The model under review builds one solid part; all positions refer to its coordinate system, in mm. A direction names the side the tool comes from. Coordinates: 2 decimals unless noted, no trailing zeros. Write each loop counter-clockwise with the first axis right and the second up, starting at its lowest first coordinate (ties: lowest second). Pieces come first, ordered by that corner, then holes. Notation, with made-up numbers: (47.5, 41) - (105.5, 41) arc R26 ccw to (105.5, 58) - close; hole circle Ø6 at (6, 86). An arc over 180 degrees is marked (long way). Return JSON: item names as keys, results as strings. Group by question number.
(1) Tool access review of faces 1 (the face through (-166.436, -12.522, 21.226)), 2 (the face through (-129, 0, 21)), 3 (the face through (-130, 0, 4)): name each direction out of +Z, -Z, +X, -X, +Y, -Y from which nothing blocks a thin tool from reaching the whole face with its end or side.
(2) To check wall thickness, follow L1, parallel to Y at x = 182, z = 10.75; L2, parallel to X at y = -7.5, z = 16.5; L3, parallel to X at y = 20, z = 4.75. State the ranges of each line that lie inside material, in increasing order. Write a range as from..to.
(3) We need section A-A on y = 12.7. State the section outline as (x, z) points.
(4) For pin 1 Ø20.5 at (x, y) = (-134, -14) entering from -Z; pin 2 Ø6 at (y, z) = (0.5, 16) entering from -X; pin 3 Ø7.5 at (x, z) = (191.5, 15) entering from -Y; pin 4 Ø5 at (x, z) = (196.67, 4.57) entering from +Y, all flat-tipped, find the tip position at first contact; note any pin that passes through.
(5) We need section C-C on y = -12.7. Give the number of separate pieces and of enclosed holes in the cut face, then the cut area to 3 significant figures.
(6) Draft analysis for pull direction Z (two halves, no side actions). For faces 4 (the face through (171.6, 12.8, 12.5)), 5 (the face through (-18, 0, 0)), 6 (the face through (-16, -25.4, 13)), 7 (the face through (-205, 0, 8.467)), state which applies: released by +Z, released by -Z, zero draft, split by the parting line, or undercut.
(7) We need section B-B on x = -136. State the section outline as (y, z) points.
```python
from build123d import *

# Parameters (mm, degrees)
F1_DEPTH  = 25.4
F3_DEPTH  = 8.4666666667
F5_DEPTH  = 8.4666666667
F6_W      = 25.4
F6_H      = 8.4666666667
F9_W      = 27.051
F9_H      = 8.4666666667
F13_R     = 6.35
F14_DEPTH = 16.9343333333
F12_R     = 3.175
F15_DEPTH = 42.3343333333
F16_R     = 6.35
F17_DEPTH = 25.401


with BuildPart() as f1:
    # F0 (on Top) → F1 (new body)
    with BuildSketch(Plane.XY):
        Polygon((-232.5293936748, 25.4), (-203.2, -25.4), (203.2, -25.4), (203.2, 25.4), align=None)
    extrude(amount=F1_DEPTH)

    # F2 (on face) → F3 (cut)
    with BuildSketch(Plane.XY.offset(25.4)):
        Polygon((-159.2059094878, 0), (-173.8706063252, -25.4), (-115.2118189755, -25.4), (-100.5471221381, 0), align=None)
    extrude(amount=-F3_DEPTH, mode=Mode.SUBTRACT)

    # F4 (on face) → F5 (cut)
    with BuildSketch(Plane(origin=(0, 0, 0), x_dir=(1, 0, 0), z_dir=(0, 0, -1))):
        Polygon((-100.5471221381, 0), (-115.2118189755, 25.4), (-173.8706063252, 25.4), (-159.2059094878, 0), align=None)
    extrude(amount=-F5_DEPTH, mode=Mode.SUBTRACT)

    # F7: sweep along a path in F7_path
    with BuildLine(Plane(origin=(-232.5293936748, 25.4, 25.4), x_dir=(-0.5, 0.8660254038, 0), z_dir=(-0.8660254038, -0.5, 0))) as f7_path:
        Line((0, 0), (-58.6587873497, 0))
    # F6 (on face) → F7 (sweep, cut)
    with BuildSketch(Plane(origin=(0, 25.4, 0), x_dir=(-1, 0, 0), z_dir=(0, 1, 0))):
        with Locations((219.8293936748, 12.7)):
            Rectangle(F6_W, F6_H)
    sweep(path=f7_path.line, mode=Mode.SUBTRACT)

    # F10: sweep along a path in F8
    with BuildLine(Plane.XZ.offset(25.4)) as f10_path:
        Line((193.9551560496, 25.4), (203.2, 0))
    # F9 (on face) → F10 (sweep, cut)
    with BuildSketch(Plane.XY.offset(25.4)):
        with Locations((180.4296560496, -21.1666666667)):
            Rectangle(F9_W, F9_H)
        with Locations((180.4296560496, -4.2333333333)):
            Rectangle(F9_W, F9_H)
        with Locations((180.4296560496, 12.7)):
            Rectangle(F9_W, F9_H)
        Polygon((203.2, 25.4), (193.9551560496, 25.4), (193.9551560496, 16.9333333333), (193.9551560496, 8.4666666667), (193.9551560496, 0), (193.9551560496, -8.4666666667), (193.9551560496, -16.9333333333), (193.9551560496, -25.4), (203.2, -25.4), align=None)
    sweep(path=f10_path.line, mode=Mode.SUBTRACT)

    # F13 (on face) → F14 (cut, through all)
    with BuildSketch(Plane.XY.offset(16.9333333333)):
        with Locations((-151.873561069, -12.7)):
            Circle(F13_R)
        with Locations((-122.5441673942, -12.7)):
            Circle(F13_R)
    extrude(amount=-F14_DEPTH, mode=Mode.SUBTRACT)

    # F12 (on face) → F15 (cut, through all)
    with BuildSketch(Plane.XZ.offset(16.9333333333)):
        with Locations((190.7538071849, 20.828)):
            Circle(F12_R)
        with Locations((196.6705073132, 4.572)):
            Circle(F12_R)
        with Locations((173.4336487365, 20.828)):
            Circle(F12_R)
        with Locations((179.3503488647, 4.572)):
            Circle(F12_R)
    extrude(amount=-F15_DEPTH, mode=Mode.SUBTRACT)

    # F16 (on face) → F17 (cut, through all)
    with BuildSketch(Plane(origin=(0, 0, 0), x_dir=(1, 0, 0), z_dir=(0, 0, -1))):
        with Locations((-195.8676515813, 12.7)):
            Circle(F16_R)
        with Locations((-210.5323484187, -12.7)):
            Circle(F16_R)
    extrude(amount=-F17_DEPTH, mode=Mode.SUBTRACT)


solid = f1.part
```
Ans:
{
 "1": {"face 1": "+Z, -Y", "face 2": "+Z", "face 3": "-Z"},
 "2": {"L1": "-16.93..-8.47, 0..8.47, 16.93..25.4", "L2": "-188.13..-155.52, -148.23..-126.19, -118.9..170.14", "L3": "-229.41..176.18, 182.52..193.5, 199.84..201.47"},
 "3": {"outline": "(-225.2, 0) - (-216.88, 0) - (-216.88, 8.47) - (-225.2, 8.47) - close; (-225.2, 16.93) - (-216.88, 16.93) - (-216.88, 25.4) - (-225.2, 25.4) - close; (-204.18, 0) - (176.15, 0) - (166.9, 25.4) - (-204.18, 25.4) - (-204.18, 16.93) - (-199.8, 16.93) - (-199.8, 8.47) - (-204.18, 8.47) - close"},
 "4": {"pin 1": "z = 8.47", "pin 2": "x = -219.8", "pin 3": "y = -16.93", "pin 4": "through"},
 "5": {"separate pieces": "5", "enclosed holes": "4", "area": "8,630 mm²"},
 "6": {"face 4": "released by +Z", "face 5": "released by -Z", "face 6": "zero draft", "face 7": "undercut"},
 "7": {"outline": "(-25.4, 8.47) - (0, 8.47) - (0, 0) - (25.4, 0) - (25.4, 25.4) - (0, 25.4) - (0, 16.93) - (-25.4, 16.93) - close"}
}
